Input: part model. Units: mm. Frame: model coordinates. A direction names the side the tool comes from. Round coordinates to 2 decimals unless told otherwise and drop trailing zeros. Write each loop counter-clockwise with the first axis right and the second up, starting at its lowest first coordinate (ties: lowest second). Pieces come first, ordered by that corner, then holes. Notation, with made-up numbers: M 80.5,71 L 103.5,71 A15 ccw 103.5,76 Z; hole C -11,82.5 d6. An arc over 180 degrees is marked long. Answer as CSV lines item,"result". Start each with the question number.
```python
from build123d import *

# Parameters (mm, degrees)
SKETCH1_R           = 3
SKETCH1_R_2         = 2
BOSS_EXTRUDE1_DEPTH = 5
SKETCH2_W           = 60
SKETCH2_H           = 7
BOSS_EXTRUDE2_DEPTH = 40
BOSS_EXTRUDE3_DEPTH = 9
SKETCH4_R           = 2.25
CUT_EXTRUDE1_DEPTH  = 8


with BuildPart() as part:
    # Sketch1 → Boss-Extrude1 (new body)
    with BuildSketch(Plane.XY):
        with BuildLine():
            Line((-30, 26.6), (-30, -25))
            Line((-30, -25), (30, -25))
            Line((30, -25), (30, 26.6))
            ThreePointArc((30, 26.6), (0, 56.6), (-30, 26.6))
        make_face()
        with Locations((0, 26.6)):
            Circle(SKETCH1_R, mode=Mode.SUBTRACT)
        with Locations((0, 40.6)):
            Circle(SKETCH1_R_2, mode=Mode.SUBTRACT)
        with Locations((0, 12.6)):
            Circle(SKETCH1_R_2, mode=Mode.SUBTRACT)
    extrude(amount=BOSS_EXTRUDE1_DEPTH)

    # Sketch2 → Boss-Extrude2 (add)
    with BuildSketch(Plane.XY.offset(5)):
        with Locations((0, -21.5)):
            Rectangle(SKETCH2_W, SKETCH2_H)
    extrude(amount=BOSS_EXTRUDE2_DEPTH)

    # Sketch3 → Boss-Extrude3 (add)
    with BuildSketch(Plane.ZY.offset(30)):
        Polygon((5, 26.6), (25, -18), (5, -18), align=None)
    boss_extrude3 = extrude(amount=-BOSS_EXTRUDE3_DEPTH)

    # Mirror1: Boss-Extrude3 across plane
    add(boss_extrude3.mirror(Plane(origin=(0, 0, 0), x_dir=(0, 0, 1), z_dir=(1, 0, 0))))

    # Sketch4 → Cut-Extrude1 (cut, through all)
    with BuildSketch(Plane(origin=(0, -18, 0), x_dir=(1, 0, 0), z_dir=(0, 1, 0))):
        with Locations(Location((16, -38, 0), (0, 0, 270))):  # turned: the seam where the file's is
            Circle(SKETCH4_R)
        with Locations(Location((-16, -38, 0), (0, 0, 270))):  # turned: the seam where the file's is
            Circle(SKETCH4_R)
        with Locations(Location((-16, -12, 0), (0, 0, 270))):  # turned: the seam where the file's is
            Circle(SKETCH4_R)
        with Locations(Location((16, -12, 0), (0, 0, 270))):  # turned: the seam where the file's is
            Circle(SKETCH4_R)
    extrude(amount=-CUT_EXTRUDE1_DEPTH, mode=Mode.SUBTRACT)


solid = part.part
```
Item 1: Pin query (flat end, axial travel): pin 1 Ø1.5 at (x, z) = (-20.5, 40) entering from +Y; pin 2 Ø1 at (x, y) = (-7.5, 44.5) entering from +Z. Return the tip coordinate at first contact, or that it passes through.
Item 2: Line query: line 1 (X direction, y = -23.25, z = 12); line 2 (X direction, y = 12.5, z = 7); line 3 (Z direction, x = 10, y = 37.5). Output: solid intervals per line, ascending. Write a range as [from, to].
Item 3: Cut plane B-B, the plane x = 0. Return loops of the section in (y, z), plus the area to 3 significant figures.
Item 4: Cut plane D-D, the plane z = 19. Return loops of the section in (x, y), plus the area to 3 significant figures.
Item 5: Cut plane A-A, the plane z = 38. Return loops of the section in (x, y), plus the area to 3 significant figures.
Item 6: Access query for faces 1 (the face through (30, -5, 13)), 2 (the face through (-21, -5, 11)). Directions: +Z, -Z, +X, -X, +Y, -Y. A direction counts if a zero-diameter tool reaches every point of the face in a straight line with its end or side. Return the directions, or none.
Item 7: Draft query along Y for faces 3 (the face through (-0.65, 23.67, 2.46)), 4 (the face through (0.923, 38.826, 2.465)), 5 (the face through (-25.56, 4.61, 14.86)), 6 (the face through (-17.996, -21.451, 39.038)). Return one class per face: +Y half, -Y half, draft (parallel to the pull), parting line (faces both ways), or undercut.
Item 8: Cut plane C-C, the plane y = 40.6. Return loops of the section in (x, z), plus the area to 3 significant figures.
Results list:
1,pin 1,"y = -18"
1,pin 2,"z = 5"
2,line 1,"[-30, -18.25], [-13.75, 13.75], [18.25, 30]"
2,line 2,"[-30, -21], [21, 30]"
2,line 3,"[0, 5]"
3,outline,"M -25,0 L 10.6,0 L 10.6,5 L -18,5 L -18,45 L -25,45 Z; M 14.6,0 L 23.6,0 L 23.6,5 L 14.6,5 Z; M 29.6,0 L 38.6,0 L 38.6,5 L 29.6,5 Z; M 42.6,0 L 56.6,0 L 56.6,5 L 42.6,5 Z"
3,area,"618 mm²"
4,outline,"M -30,-25 L 30,-25 L 30,-4.62 L 21,-4.62 L 21,-18 L -21,-18 L -21,-4.62 L -30,-4.62 Z"
4,area,"661 mm²"
5,outline,"M -30,-25 L -18.25,-25 L -18.25,-18 L -30,-18 Z; M -13.75,-25 L 13.75,-25 L 13.75,-18 L -13.75,-18 Z; M 18.25,-25 L 30,-25 L 30,-18 L 18.25,-18 Z"
5,area,"357 mm²"
6,face 1,"+Z, -Z, +X, +Y, -Y"
6,face 2,"+Z, +Y"
7,face 3,"undercut"
7,face 4,"undercut"
7,face 5,"+Y half"
7,face 6,"draft"
8,outline,"M -26.53,0 L -2,0 L -2,5 L -26.53,5 Z; M 2,0 L 26.53,0 L 26.53,5 L 2,5 Z"
8,area,"245 mm²"
